Answer from the drawing. Dimensions are ordinates in mm from the lowest x, y and z of the part. A direction names the side the tool comes from. Give positions to 0.01 mm unless a question says otherwise; leave off trailing zeros. Write each loop counter-clockwise with the first axis right and the second up, starting at its lowest first coordinate (ties: lowest second). Pieces come first, ordered by that corner, then holes. Notation, with made-up numbers: (25.5, 8.25) -> (35.5, 8.25) arc R22 ccw to (35.5, 17.25) -> close; hole circle Ø10 at (57.5, 11.5). An arc over 180 degrees is marked (long way). Put each result on its own line as item: value. Start each with the question number.
1) For a pull along Y with two mould halves and no side action, classify the marked faces 1, 2, 3 and 4 as released by +Y, released by -Y, zero draft, split by the parting line, or undercut.
2) Flat-ended cylindrical pins translate along their axes: pin 1 Ø1.5 at (y, z) = (26, 2.5) entering from +X; pin 2 Ø4 at (x, z) = (22.5, 7) entering from -Y; pin 3 Ø2 at (x, z) = (24.5, 6.5) entering from -Y. Find the tip coordinate at first contact, or state that the pin passes through.
3) A cutting plane is placed at D-D (y = 22). Write down the section's boundary in (x, z), then the cut area to 3 significant figures.
4) A cutting plane is placed at C-C (z = 9.5). Write down the section's boundary in (x, y).
5) For the marked faces 5 and 6, determine the directions among +Z, -Z, +X, -X, +Y, -Y from which every point of the face is accessible in a straight line to the end or side of a thin tool.
6) Find the intervals of material crossed by line 1 along Y through (x, z) = (15, 8.7); line 2 along Y through (x, z) = (15, 4.5); line 3 along Y through (x, z) = (12.75, 9.25), in increasing order. Write a range as from..to.
7) A cutting plane is placed at A-A (x = 15). Write down the section's boundary in (y, z), then the cut area to 3 significant figures.
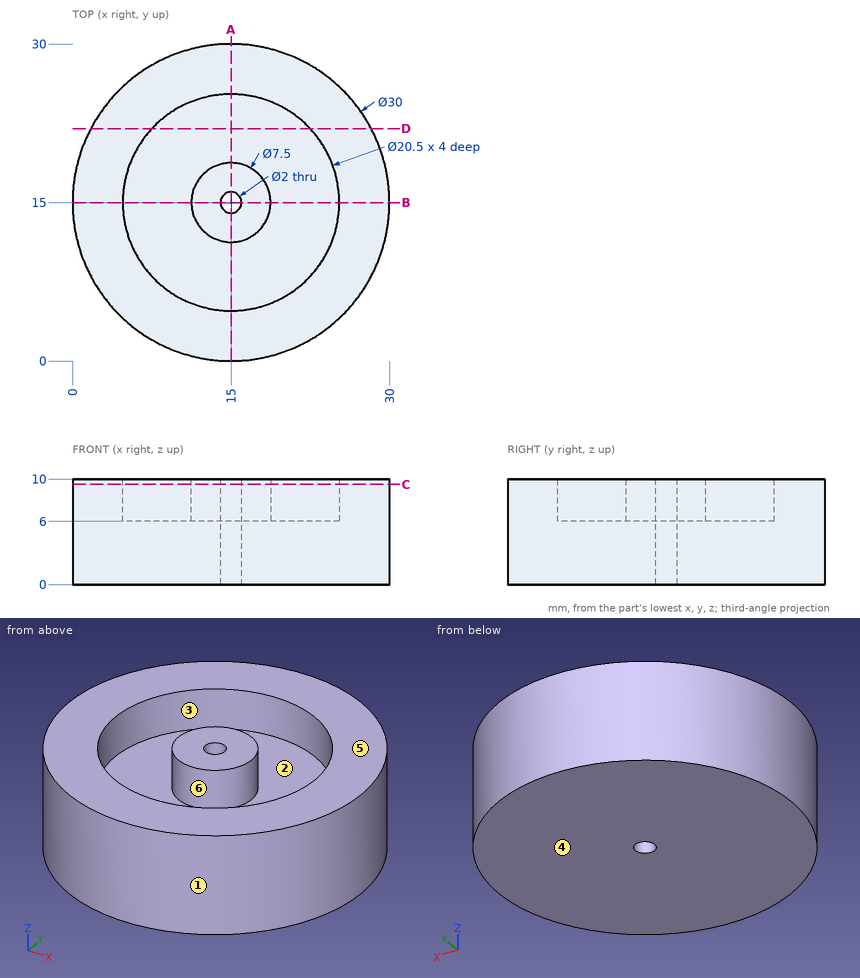
Reply:
1. face 1: split by the parting line
1. face 2: undercut
1. face 3: undercut
1. face 4: zero draft
2. pin 1: stops at x = 25.95
2. pin 2: stops at y = 1.04
2. pin 3: stops at y = 2.64
3. outline: (1.73, 0) -> (28.27, 0) -> (28.27, 10) -> (22.49, 10) -> (22.49, 6) -> (7.51, 6) -> (7.51, 10) -> (1.73, 10) -> close
3. area: 205 mm2
4. outline: circle Ø30 at (15, 15); circle Ø7.5 at (15, 15); hole circle Ø20.5 at (15, 15); hole circle Ø2 at (15, 15)
5. face 5: +Z, +X, -X, +Y, -Y
5. face 6: +Z
6. line 1: y = 0..4.75, 11.25..14, 16..18.75, 25.25..30
6. line 2: y = 0..14, 16..30
6. line 3: y = 0.17..5, 12..18, 25..29.83
7. outline: (0, 0) -> (14, 0) -> (14, 10) -> (11.25, 10) -> (11.25, 6) -> (4.75, 6) -> (4.75, 10) -> (0, 10) -> close; (16, 0) -> (30, 0) -> (30, 10) -> (25.25, 10) -> (25.25, 6) -> (18.75, 6) -> (18.75, 10) -> (16, 10) -> close
7. area: 228 mm2
